Design review of the part built by this model. Coordinates are the model's own, in mm. Coordinates: 2 decimals unless noted, no trailing zeros. Loops run counter-clockwise (first coordinate to the right, second up) from the corner with the lowest first, then second, coordinate; pieces in that order, holes last. Notation, with made-up numbers: (-5.5, 13.25) - (32.5, 13.25) arc R24 cw to (32.5, 33.25) - close; hole circle Ø5 at (31.25, 65.5). An arc over 180 degrees is marked (long way). Answer in a Markdown table with one row per item. Add a question column.
(1) Clearance check with flat-ended pins moving along their axes: pin 1 (6 mm diameter, centred on y = 2, z = -3.5, fed in from +X); pin 2 (2.5 mm diameter, centred on x = -21.3, z = 14.24, fed in from +Y); pin 3 (1 mm diameter, centred on x = 0.5, y = 4.5, fed in from -Z); pin 4 (3 mm diameter, centred on y = 5.5, z = -28, fed in from +X). State where each tip first meets the part, or that it passes through.
(2) We need section D-D, the plane z = 13.5. Write out the cut boundary in (x, y), plus the area to 3 significant figures.
(3) To check wall thickness, follow L1, parallel to Z at x = 14, y = 4.5; L2, parallel to Z at x = -1, y = 5.5; L3, parallel to X at y = 3, z = 13. State the ranges of each line that lie inside material, in increasing order. Write a range as [from, to].
(4) The part is to be moulded in two halves that separate along X. For faces 1 (the face through (15.07, 4.93, -3.35)), 2 (the face through (-14.514, 4.93, -9.604)), 3 (the face through (2, 0, -1)), say which applies: released by +X, released by -X, zero draft, split by the parting line, or undercut.
(5) We need section A-A, the plane x = 8. Write out the cut boundary in (y, z), plus the area to 3 significant figures.
(6) We need section C-C, the plane y = 5.25. Write out the cut boundary in (x, z).
(7) We need section B-B, the plane z = -19. Write out the cut boundary in (x, y), plus the area to 3 significant figures.
from build123d import *

# Parameters (mm, degrees)
SKETCH1_R           = 2.070000001
SKETCH1_R_2         = 2.07
SKETCH1_R_3         = 6.5
BOSS_EXTRUDE1_DEPTH = 10


with BuildPart() as part:
    # Sketch1 → Boss-Extrude1 (new body)
    with BuildSketch(Plane(origin=(0, 0, 0), x_dir=(1, 0, 0), z_dir=(0, 1, 0))):
        with BuildLine():
            Line((23.703500556, -15.152403716), (23.64205667, 15.828297469))
            ThreePointArc((23.64205667, 15.828297469), (23.296182467, 18.41580704), (22.292396885, 20.825630528))
            Line((22.292396885, 20.825630528), (13.99606221, 35.129712685))
            ThreePointArc((13.99606221, 35.129712685), (0.385615186, 40.666219429), (-8.382044752, 28.875319789))
            ThreePointArc((-8.382044752, 28.875319789), (-9.316904265, 20.837743246), (-12.365890121, 13.342392404))
            Line((-12.365890121, 13.342392404), (-16.723498541, 5.760104356))
            ThreePointArc((-16.723498541, 5.760104356), (-21.220226961, -0.19980824), (-27.049399397, -4.864770548))
            ThreePointArc((-27.049399397, -4.864770548), (-31.881873053, -17.239982686), (-21.276578026, -25.241632171))
            Line((-21.276578026, -25.241632171), (13.723353139, -25.172216965))
            ThreePointArc((13.723353139, -25.172216965), (20.788598117, -22.229266547), (23.703500556, -15.152403716))
        make_face()
        with Locations(Location((-21.298394234, -14.241653805, 0), (0, 0, 270))):
            Circle(SKETCH1_R, mode=Mode.SUBTRACT)
        with Locations(Location((-1.298433568, -14.201987971, 0), (0, 0, 270))):
            Circle(SKETCH1_R_2, mode=Mode.SUBTRACT)
        with Locations(Location((13.69955364, -13.172240563, 0), (0, 0, 270))):
            Circle(SKETCH1_R_2, mode=Mode.SUBTRACT)
        with Locations(Location((13.669804266, 1.827729936, 0), (0, 0, 270))):
            Circle(SKETCH1_R_2, mode=Mode.SUBTRACT)
        with Locations(Location((3.615677553, 19.807825031, 0), (0, 0, 270))):
            Circle(SKETCH1_R_3, mode=Mode.SUBTRACT)
    extrude(amount=BOSS_EXTRUDE1_DEPTH)


solid = part.part
Responses:
| question | item | result |
|---|---|---|
| 1 | pin 1 | stops at x = 23.67 |
| 1 | pin 2 | passes through |
| 1 | pin 3 | stops at z = -40.82 |
| 1 | pin 4 | stops at x = 19 |
| 2 | outline | (-32.27, 0) - (-23.23, 0) - (-23.23, 10) - (-32.27, 10) - close; (-19.37, 0) - (-3.25, 0) - (-3.25, 10) - (-19.37, 10) - close; (0.65, 0) - (11.66, 0) - (11.66, 10) - (0.65, 10) - close; (15.74, 0) - (23.7, 0) - (23.7, 10) - (15.74, 10) - close |
| 2 | area | 441 mm2 |
| 3 | L1 | z = [-35.12, -3.87], [0.22, 11.12], [15.22, 25.17] |
| 3 | L2 | z = [-40.19, -24.38], [-15.23, 12.15], [16.25, 25.2] |
| 3 | L3 | x = [-32.23, -22.95], [-19.64, -2.98], [0.39, 11.64], [15.76, 23.7] |
| 4 | face 1 | undercut |
| 4 | face 2 | released by -X |
| 4 | face 3 | zero draft |
| 5 | outline | (0, -40.28) - (10, -40.28) - (10, -24.61) - (0, -24.61) - close; (0, -15.01) - (10, -15.01) - (10, 25.18) - (0, 25.18) - close |
| 5 | area | 559 mm2 |
| 6 | outline | (-27.05, 4.86) arc R30 cw to (-16.72, -5.76) - (-12.37, -13.34) arc R30 cw to (-8.38, -28.88) arc R12 ccw to (14, -35.13) - (22.29, -20.83) arc R10 ccw to (23.64, -15.83) - (23.7, 15.15) arc R10 ccw to (13.72, 25.17) - (-21.28, 25.24) arc R11 ccw to start; hole circle Ø4.14 at (-21.3, 14.24); hole circle Ø4.14 at (-1.3, 14.2); hole circle Ø13 at (3.62, -19.81); hole circle Ø4.14 at (13.67, -1.83); hole circle Ø4.14 at (13.7, 13.17) |
| 7 | outline | (-9.85, 0) - (-2.83, 0) - (-2.83, 10) - (-9.85, 10) - close; (10.07, 0) - (23.12, 0) - (23.12, 10) - (10.07, 10) - close |
| 7 | area | 201 mm2 |
